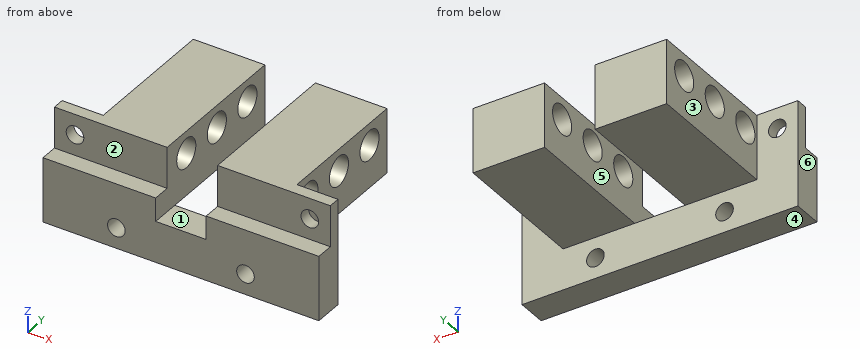
```python
from build123d import *

# Parameters (mm, degrees)
BOSS_EXTRUDE1_DEPTH = 11
CUT_EXTRUDE1_REACH  = 37.52
SKETCH3_W           = 7
SKETCH3_H           = 3
CUT_EXTRUDE2_REACH  = 34.538
SKETCH4_R           = 2.5
SKETCH5_R           = 1.5
CUT_EXTRUDE3_DEPTH  = 11
SKETCH6_W           = 47
SKETCH6_H           = 5
BOSS_EXTRUDE2_DEPTH = 7
SKETCH7_R           = 1.5
CUT_EXTRUDE4_DEPTH  = 5
SKETCH9_R           = 2.5
BOSS_EXTRUDE3_DEPTH = 1.2
SKETCH10_R          = 2.5
BOSS_EXTRUDE4_DEPTH = 1.2


with BuildPart() as part:
    # Sketch1 → Boss-Extrude1 (new body)
    with BuildSketch(Plane.XY):
        Polygon((0, 0), (18, 0), (18, 28.578), (7, 28.578), (7, 5), (0, 5), align=None)
    extrude(amount=BOSS_EXTRUDE1_DEPTH)

    # Sketch3 → Cut-Extrude1 (cut, up to next)
    with BuildSketch(Plane.ZY, mode=Mode.PRIVATE) as cut_extrude1_sk1:
        with Locations((7.5, 1.5)):
            Rectangle(SKETCH3_W, SKETCH3_H)
    cut_extrude1_tool1 = extrude(cut_extrude1_sk1.sketch, amount=-CUT_EXTRUDE1_REACH, mode=Mode.PRIVATE) & part.part
    add(cut_extrude1_tool1.solids().sort_by_distance((0, 1.5, 7.5))[0], mode=Mode.SUBTRACT)

    # Sketch4 → Cut-Extrude2 (cut, up to next)
    with BuildSketch(Plane.ZY.offset(-7), mode=Mode.PRIVATE) as cut_extrude2_sk1:
        with Locations(Location((7.25, 8, 0), (0, 0, 270))):
            Circle(SKETCH4_R)
    cut_extrude2_tool1 = extrude(cut_extrude2_sk1.sketch, amount=-CUT_EXTRUDE2_REACH, mode=Mode.PRIVATE) & part.part
    # Sketch4 → Cut-Extrude2 (cut, up to next)
    with BuildSketch(Plane.ZY.offset(-7), mode=Mode.PRIVATE) as cut_extrude2_sk2:
        with Locations(Location((7.25, 16, 0), (0, 0, 270))):
            Circle(SKETCH4_R)
    cut_extrude2_tool2 = extrude(cut_extrude2_sk2.sketch, amount=-CUT_EXTRUDE2_REACH, mode=Mode.PRIVATE) & part.part
    # Sketch4 → Cut-Extrude2 (cut, up to next)
    with BuildSketch(Plane.ZY.offset(-7), mode=Mode.PRIVATE) as cut_extrude2_sk3:
        with Locations(Location((7.25, 24, 0), (0, 0, 270))):
            Circle(SKETCH4_R)
    cut_extrude2_tool3 = extrude(cut_extrude2_sk3.sketch, amount=-CUT_EXTRUDE2_REACH, mode=Mode.PRIVATE) & part.part
    add(cut_extrude2_tool1.solids().sort_by_distance((7, 8, 7.25))[0], mode=Mode.SUBTRACT)
    add(cut_extrude2_tool2.solids().sort_by_distance((7, 16, 7.25))[0], mode=Mode.SUBTRACT)
    add(cut_extrude2_tool3.solids().sort_by_distance((7, 24, 7.25))[0], mode=Mode.SUBTRACT)

    # Sketch5 → Cut-Extrude3 (cut)
    with BuildSketch(Plane(origin=(0, 5, 0), x_dir=(1, 0, 0), z_dir=(0, 1, 0))):
        with Locations(Location((3.5, -7.5, 0), (0, 0, 180))):
            Circle(SKETCH5_R)
    extrude(amount=-CUT_EXTRUDE3_DEPTH, mode=Mode.SUBTRACT)


with BuildPart() as body_2:
    # Mirror6: mirrored copy
    add(part.part.mirror(Plane(origin=(23.5, 0, 0), x_dir=(0, 0, 1), z_dir=(1, 0, 0))))


with BuildPart() as part_1:
    add(part.part)

    add(body_2.part)  # Boss-Extrude2 merges body 2
    # Sketch6 → Boss-Extrude2 (add)
    with BuildSketch(Plane(origin=(0, 0, 0), x_dir=(-1, 0, 0), z_dir=(0, 0, -1))):
        with Locations((-23.5, 2.5)):
            Rectangle(SKETCH6_W, SKETCH6_H)
    extrude(amount=BOSS_EXTRUDE2_DEPTH)

    # Sketch7 → Cut-Extrude4 (cut)
    with BuildSketch(Plane(origin=(0, 5, 0), x_dir=(1, 0, 0), z_dir=(0, 1, 0))):
        with Locations(Location((12.5, 3.5, 0), (0, 0, 180))):
            Circle(SKETCH7_R)
        with Locations(Location((34.5, 3.5, 0), (0, 0, 270))):
            Circle(SKETCH7_R)
    extrude(amount=-CUT_EXTRUDE4_DEPTH, mode=Mode.SUBTRACT)

    # Sketch9 → Boss-Extrude3 (add)
    with BuildSketch(Plane.ZY.offset(-29)):
        Polygon((11, 3), (11, 28.578), (0, 28.578), (0, 5), (0, 0), (4, 0), (4, 3), align=None)
        with Locations(Location((7.25, 24, 0), (0, 0, 270))):
            Circle(SKETCH9_R, mode=Mode.SUBTRACT)
        with Locations(Location((7.25, 16, 0), (0, 0, 270))):
            Circle(SKETCH9_R, mode=Mode.SUBTRACT)
        with Locations(Location((7.25, 8, 0), (0, 0, 270))):
            Circle(SKETCH9_R, mode=Mode.SUBTRACT)
    extrude(amount=BOSS_EXTRUDE3_DEPTH)

    # Sketch10 → Boss-Extrude4 (add)
    with BuildSketch(Plane(origin=(18, 0, 0), x_dir=(0, 0, -1), z_dir=(1, 0, 0))):
        Polygon((-11, 28.578), (-11, 3), (-4, 3), (-4, 0), (0, 0), (0, 5), (0, 28.578), align=None)
        with Locations(Location((-7.25, 8, 0), (0, 0, 270))):
            Circle(SKETCH10_R, mode=Mode.SUBTRACT)
        with Locations(Location((-7.25, 16, 0), (0, 0, 270))):
            Circle(SKETCH10_R, mode=Mode.SUBTRACT)
        with Locations(Location((-7.25, 24, 0), (0, 0, 270))):
            Circle(SKETCH10_R, mode=Mode.SUBTRACT)
    extrude(amount=BOSS_EXTRUDE4_DEPTH)


solid = part_1.part
```
Design review of the part built by this model. Coordinates are the model's own, in mm. Face numbers are marked on the shaded views. A direction names the side the tool comes from. Give positions to 0.01 mm unless a question says otherwise; leave off trailing zeros. Order: outer loops, then holes, each group sorted by start corner. A loop starts at its lowest first (then second) coordinate and runs counter-clockwise, first axis right, second up. Notation, with made-up numbers: (-7, 38) - (27, 38) arc R14 cw to (27, 48) - close; hole circle Ø9 at (-37.5, -6.75). An arc over 180 degrees is marked (long way). Use a Markdown table: item, result. Add a question column.
(1) Add section A-A on z = 1. Give the boundary of the cut face in (x, y), then the cut area to 3 significant figures.
(2) Add section B-B on y = 12.25. Give the boundary of the cut face in (x, z), then the cut area to 3 significant figures.
(3) Add section D-D on z = -3.5. Give the boundary of the cut face in (x, y), then the cut area to 3 significant figures.
(4) Wall thickness on probe 1 along Y at (x, z) = (15, 7.25); probe 2 along X at (y, z) = (3.75, 1.5); probe 3 along X at (y, z) = (19, 4): over which ranges is each line inside the solid? List them lowest first. Write a range as [from, to].
(5) Add section C-C on x = 8. Give the boundary of the cut face in (y, z).
(6) Clearance check with flat-ended pins moving along their axes: P1, Ø3.5, axis at x = 42, y = 1, coming from the +Z side; P2, Ø2.5, axis at x = 34.5, z = -3.5, coming from the -Y side; P3, Ø1, axis at x = 19, y = 7, coming from the -Z side; P4, Ø3, axis at x = 20.5, z = 9, coming from the -Y side. State where each tip first meets the part, or that it passes through.
(7) Mouldability with a two-part tool opening along X and no side actions: class the marked faces 4, 5 and 6 as +X half, -X half, draft (parallel to the pull), parting line (faces both ways), or undercut.
(8) Machinability: for the marked faces 1, 2 and 3, which of the approach directions +Z, -Z, +X, -X, +Y, -Y give a long, thin tool a straight path to every point of the face, cutting with its end or side? Answer none if there is none.
Report:
| question | item | result |
|---|---|---|
| 1 | outline | (0, 0) - (19.2, 0) - (19.2, 28.58) - (7, 28.58) - (7, 5) - (0, 5) - close; (27.8, 0) - (47, 0) - (47, 5) - (40, 5) - (40, 28.58) - (27.8, 28.58) - close |
| 1 | area | 767 mm² |
| 2 | outline | (7, 0) - (19.2, 0) - (19.2, 11) - (7, 11) - close; (27.8, 0) - (40, 0) - (40, 11) - (27.8, 11) - close |
| 2 | area | 268 mm² |
| 3 | outline | (0, 0) - (11, 0) - (11, 5) - (0, 5) - close; (14, 0) - (33, 0) - (33, 5) - (14, 5) - close; (36, 0) - (47, 0) - (47, 5) - (36, 5) - close |
| 3 | area | 205 mm² |
| 4 | probe 1 | y = [3, 5.5], [10.5, 13.5], [18.5, 21.5], [26.5, 28.58] |
| 4 | probe 2 | x = [0, 19.2], [27.8, 47] |
| 4 | probe 3 | x = [7, 19.2], [27.8, 40] |
| 5 | outline | (0, -7) - (5, -7) - (5, 0) - (28.58, 0) - (28.58, 11) - (3, 11) - (3, 4) - (0, 4) - close; hole circle Ø5 at (8, 7.25); hole circle Ø5 at (16, 7.25); hole circle Ø5 at (24, 7.25) |
| 6 | P1 | stops at z = 4 |
| 6 | P2 | passes through |
| 6 | P3 | stops at z = 0 |
| 6 | P4 | stops at y = 3 |
| 7 | face 4 | draft |
| 7 | face 5 | undercut |
| 7 | face 6 | -X half |
| 8 | face 1 | +Z, +Y, -Y |
| 8 | face 2 | +Z, +X, -X, -Y |
| 8 | face 3 | +Z, -Z, -X, +Y |
